Source: CAD feature listing. Evaluate the final solid. Frame: model axes, mm. Give positions to 0.01 mm unless a question says otherwise; leave off trailing zeros. Order: outer loops, then holes, each group sorted by start corner. A loop starts at its lowest first (then second) coordinate and runs counter-clockwise, first axis right, second up. Notation, with made-up numbers: (15, 39) - (60, 39) arc R30 ccw to (60, 71) - close; hole circle Ø2 at (58, 31.25). An arc over 180 degrees is marked (long way). One line per item, written item: value. Start each with the question number.
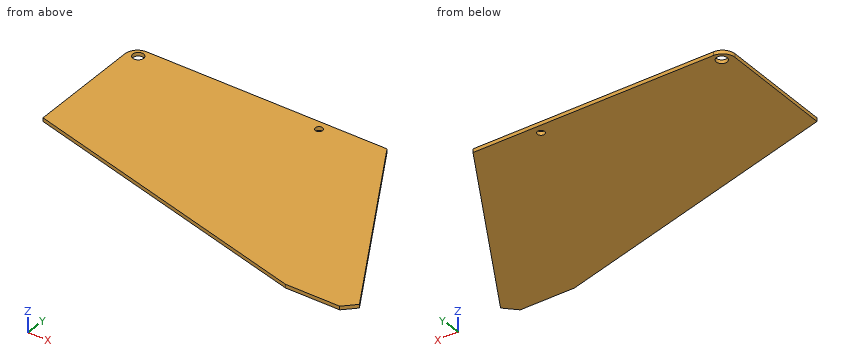
from build123d import *

# Parameters (mm, degrees)
SKETCH1_W           = 700
SKETCH1_H           = 350
BOSS_EXTRUDE2_DEPTH = 5
SKETCH2_R           = 15
SKETCH2_R_2         = 10
CUT_EXTRUDE1_DEPTH  = 10
FILLET1_R           = 35
CHAMFER1_SIZE       = 50
CHAMFER1_SIZE2      = 36.602540378


with BuildPart() as part:
    # Sketch1 → Boss-Extrude2 (new, symmetric)
    with BuildSketch(Plane.XY):
        Polygon((350, -175), (-350, -175), (480.560796608, -397.548094716), (680.560796608, -397.548094716), (350, 175), align=None)
        Rectangle(SKETCH1_W, SKETCH1_H)
    extrude(amount=BOSS_EXTRUDE2_DEPTH, both=True)

    # Sketch2 → Cut-Extrude1 (cut)
    with BuildSketch(Plane.XY.offset(5)):
        with Locations((-320, 150)):
            Circle(SKETCH2_R)
        with Locations((180, 150)):
            Circle(SKETCH2_R_2)
    extrude(amount=-CUT_EXTRUDE1_DEPTH, mode=Mode.SUBTRACT)

    # Fillet1
    fillet1_edges = [part.edges().sort_by_distance(p)[0] for p in [
        (-350, 175, 0),
    ]]
    fillet(fillet1_edges, radius=FILLET1_R)

    # Chamfer1
    chamfer1_edges = [part.edges().sort_by_distance(p)[0] for p in [
        (680.560796608, -397.548094716, 0),
    ]]
    chamfer1_side = [part.faces().sort_by_distance(p)[0] for p in [
        (580.560796608, -397.548094716, 0),
    ]]
    chamfer(chamfer1_edges, length=CHAMFER1_SIZE, length2=CHAMFER1_SIZE2, reference=chamfer1_side[0])


solid = part.part
1. Section D-D on y = -185. Return the cut outline in (x, z), then the cut area to 3 significant figures.
2. Section B-B on y = 150. Return the cut outline in (x, z), then the cut area to 3 significant figures.
3. Contact query for flat-ended pins moving along their axis: pin 1 Ø5 at (x, z) = (352, -2) entering from +Y; pin 2 Ø4 at (x, z) = (179, -1.5) entering from -Y. Output: stop coordinate, or through.
4. Ray query, L1, parallel to Y at x = 180, z = -1; L2, parallel to Y at x = 555, z = -2; L3, parallel to X at y = 96, z = -2. Return the intervals inside material, ascending.
5. Section A-A on z = -3.5. Return the cut outline in (x, y).
6. Section C-C on x = 180. Return the cut outline in (y, z).
Data:
1. outline: (-312.68, -5) - (557.85, -5) - (557.85, 5) - (-312.68, 5) - close
1. area: 8,710 mm2
2. outline: (-348.54, -5) - (-335, -5) - (-335, 5) - (-348.54, 5) - close; (-305, -5) - (170, -5) - (170, 5) - (-305, 5) - close; (190, -5) - (364.43, -5) - (364.43, 5) - (190, 5) - close
2. area: 6,630 mm2
3. pin 1: stops at y = 175
3. pin 2: stops at y = -317.28
4. L1: y = -317.01 to 140, 160 to 175
4. L2: y = -397.55 to -180.07
4. L3: x = -350 to 395.61
5. outline: (-350, -175) - (480.56, -397.55) - (630.56, -397.55) - (662.26, -365.85) - (350, 175) - (-315, 175) arc R35 ccw to (-350, 140) - close; hole circle Ø30 at (-320, 150); hole circle Ø20 at (180, 150)
6. outline: (-317.01, -5) - (140, -5) - (140, 5) - (-317.01, 5) - close; (160, -5) - (175, -5) - (175, 5) - (160, 5) - close
